Could you check a few things on this model? Use its own coordinates, in mm. A direction names the side the tool comes from. Give positions to 0.01 mm unless a question says otherwise; leave off trailing zeros. Order: outer loops, then holes, each group sorted by start corner. A loop starts at its lowest first (then second) coordinate and runs counter-clockwise, first axis right, second up.
from build123d import *

# Parameters (mm, degrees)
F0_R     = 11.2
F1_DEPTH = 7


with BuildPart() as f1:
    # F0 (on Front) → F1 (new body)
    with BuildSketch(Plane.XZ):
        with BuildLine():
            Line((30.609758, -2.393342), (9.231073, 17.274573))
            ThreePointArc((9.231073, 17.274573), (6.224822, 38.350085), (-12.972782, 29.148631))
            Line((-12.972782, 29.148631), (-20.007871, 0))
            ThreePointArc((-20.007871, 0), (-35.829886, -16.014885), (-14.374704, -22.833085))
            Line((-14.374704, -22.833085), (10.027457, -16.50023))
            ThreePointArc((10.027457, -16.50023), (30.218147, -23.89046), (30.609758, -2.393342))
        make_face()
        with Locations((-23.014148, -12.853105)):
            Circle(F0_R, mode=Mode.SUBTRACT)
        with Locations((22.75558, -13.002389)):
            Circle(F0_R, mode=Mode.SUBTRACT)
        Circle(F0_R, mode=Mode.SUBTRACT)
        with Locations((0, 26.71)):
            Circle(F0_R, mode=Mode.SUBTRACT)
    extrude(amount=F1_DEPTH)


solid = f1.part
Item 1: Imagine slicing it at D-D on x = 0. List the corners of the cut face in (y, z) for me, then the cut area to 3 significant figures.
Findings:
outline: (-7, -19.1) - (0, -19.1) - (0, -11.2) - (-7, -11.2) - close; (-7, 11.2) - (0, 11.2) - (0, 15.51) - (-7, 15.51) - close; (-7, 37.91) - (0, 37.91) - (0, 39.91) - (-7, 39.91) - close
area: 99.5 mm2
Item 2: For pin 1 (1 mm diameter, centred on y = -3, z = -18.5, fed in from -X); pin 2 (3 mm diameter, centred on y = -3, z = 28.5, fed in from -X); pin 3 (4 mm diameter, centred on x = -3, y = -4, fed in from -Z), each with a flat end and sliding along its axis, tell me the tip position at first contact or that it passes through.
Findings:
pin 1: stops at x = -35.17
pin 2: stops at x = -13.49
pin 3: stops at z = -20.4
Item 3: We'd pull the mould along X, two halves only. Please class faces 4 (the cylindrical face through (29.9, -3.5, -24.1)), 5 (the flat face through (0, 0, 12)), 6 (the cylindrical face through (6.5, -3.5, 38.2)): +X half, -X half, draft (parallel to the pull), parting line (faces both ways), or undercut.
Findings:
face 4: undercut
face 5: draft
face 6: parting line
Item 4: For faces 1 (the flat face through (20.07, -3.451, 7.303)), 2 (the flat face through (-2.3, -3.5, -19.7)), 3 (the cylindrical face through (-35.915, -3.451, -15.647)), which set-ups out of +Z, -Z, +X, -X, +Y, -Y let a thin tool reach every point of the face, with its end or its side?
Findings:
face 1: +X, +Y, -Y
face 2: -Z, +Y, -Y
face 3: +Y, -Y
Item 5: Imagine slicing it at A-A on x = 26. List the corners of the cut face in (y, z) for me, then the cut area to 3 significant figures.
Findings:
outline: (-7, -25.8) - (0, -25.8) - (0, -23.72) - (-7, -23.72) - close; (-7, -2.28) - (0, -2.28) - (0, 1.85) - (-7, 1.85) - close
area: 43.4 mm2
Item 6: Imagine slicing it at B-B on z = 26.71. List the corners of the cut face in (x, y) for me.
Findings:
outline: (-13.56, -7) - (-11.2, -7) - (-11.2, 0) - (-13.56, 0) - close; (11.2, -7) - (13.2, -7) - (13.2, 0) - (11.2, 0) - close
Item 7: Imagine slicing it at C-C on y = -5.5. List the corners of the cut face in (x, z) for me, then the cut area to 3 significant figures.
Findings:
outline: (-20.01, 0) arc R13.2 ccw (long way) to (-14.37, -22.83) - (10.03, -16.5) arc R13.2 ccw (long way) to (30.61, -2.39) - (9.23, 17.27) arc R13.2 ccw (long way) to (-12.97, 29.15) - close; hole circle Ø22.4 at (-23.01, -12.85); hole circle Ø22.4 at (0, 0); hole circle Ø22.4 at (0, 26.71); hole circle Ø22.4 at (22.76, -13)
area: 1,130 mm2
Item 8: Please list where these lines run through material, in increasing order: line 1 along X through (y, z) = (-2.25, -12.5); line 2 along Z through (x, y) = (0, -4.75); line 3 along Z through (x, y) = (-9.5, -3.25).
Findings:
line 1: x = -36.21 to -34.21, -11.82 to 11.57, 33.94 to 35.95
line 2: z = -19.1 to -11.2, 11.2 to 15.51, 37.91 to 39.91
line 3: z = -21.57 to -5.93, 5.93 to 20.78, 32.64 to 35.87
